Check sheet for the drawn part. Datum: minimum x, y, z corner. Units: mm. Coordinates: 2 decimals unless noted, no trailing zeros. Loops run counter-clockwise (first coordinate to the right, second up) from the corner with the lowest first, then second, coordinate; pieces in that order, holes last.
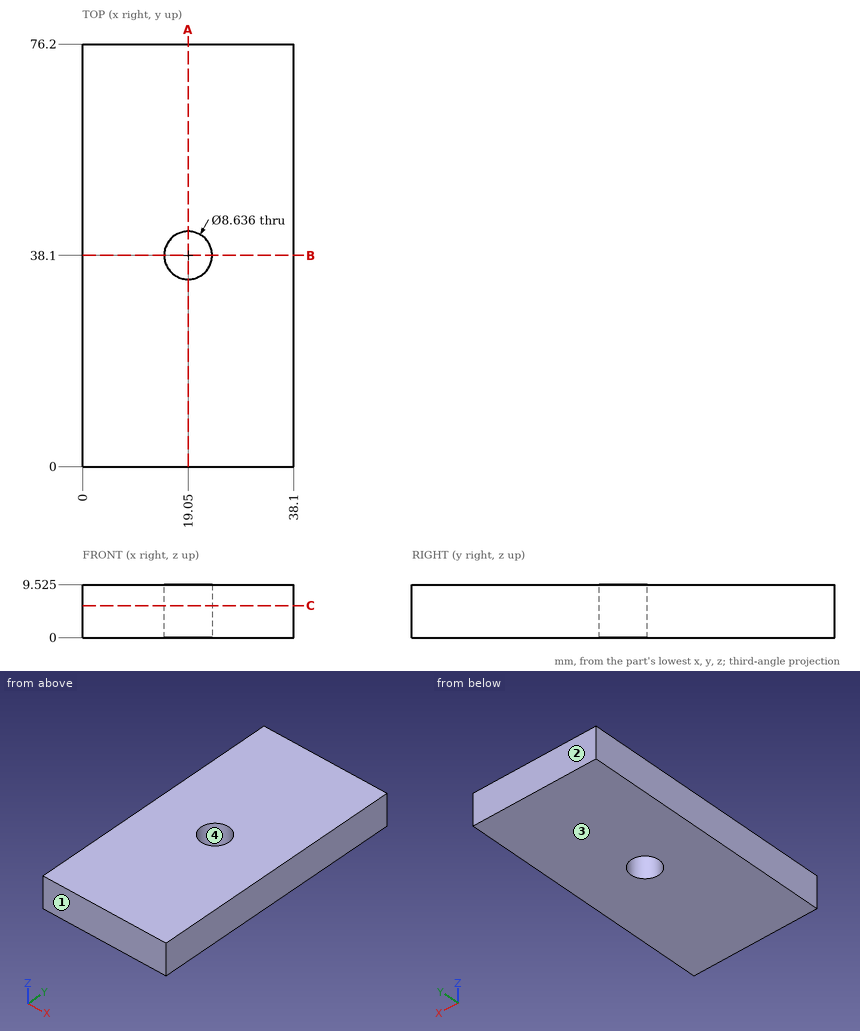
1) Mould release check, pull along Y, two halves, no side actions. Record for the marked faces 1, 2, 3 and 4: +Y half, -Y half, draft (parallel to the pull), parting line (faces both ways), or undercut.
Answer sheet:
face 1: -Y half
face 2: +Y half
face 3: draft
face 4: undercut
2) Section check A-A on x = 19.05. Enter the section's corners in (y, z) (3 decimals).
Answer sheet:
outline: (0, 0) - (33.782, 0) - (33.782, 9.525) - (0, 9.525) - close; (42.418, 0) - (76.2, 0) - (76.2, 9.525) - (42.418, 9.525) - close
3) Section check C-C on z = 5.75. Enter the section's corners in (x, y).
Answer sheet:
outline: (0, 0) - (38.1, 0) - (38.1, 76.2) - (0, 76.2) - close; hole circle Ø8.64 at (19.05, 38.1)
4) Section check B-B on y = 38.1. Enter the section's corners in (x, z) (3 decimals).
Answer sheet:
outline: (0, 0) - (14.732, 0) - (14.732, 9.525) - (0, 9.525) - close; (23.368, 0) - (38.1, 0) - (38.1, 9.525) - (23.368, 9.525) - close
5) Scan lines: line 1 (Y direction, x = 19.05, z = 6.75); line 2 (Y direction, x = 16.5, z = 8). Record each from-to range of solid material in increasing order.
Answer sheet:
line 1: y = 0 to 33.78, 42.42 to 76.2
line 2: y = 0 to 34.62, 41.58 to 76.2
